Verification items for this drawing (mm, ordinates from the low corner). Round coordinates to 2 decimals unless told otherwise and drop trailing zeros. Write each loop counter-clockwise with the first axis right and the second up, starting at its lowest first coordinate (ties: lowest second). Pieces come first, ordered by that corner, then holes.
Item 1: Cross-section at A-A (x = 8). Enter the section's corners in (y, z).
Item 2: Scan lines: probe 1 along Y at (x, z) = (15.5, 3.5); probe 2 along Z at (x, y) = (17.5, 7.5) (1 decimal); probe 3 along Y at (x, z) = (12.5, 5.75). Record each from-to range of solid material in increasing order.
Item 3: Depth check by flat-ended pin: P1, Ø2, axis at y = 6, z = 3.5, coming from the -X side; P2, Ø1.5, axis at x = 22.5, z = 5, coming from the -Y side; P3, Ø2, axis at x = 14, z = 1.5, coming from the +Y side. Enter the tip coordinate at first touch or a pass-through.
Item 4: Draft check along Z on the marked faces 1 and 2. Enter one of: pulls with the +Z half, pulls with the -Z half, needs draft (parallel to the pull), parting line crosses it, or undercut.
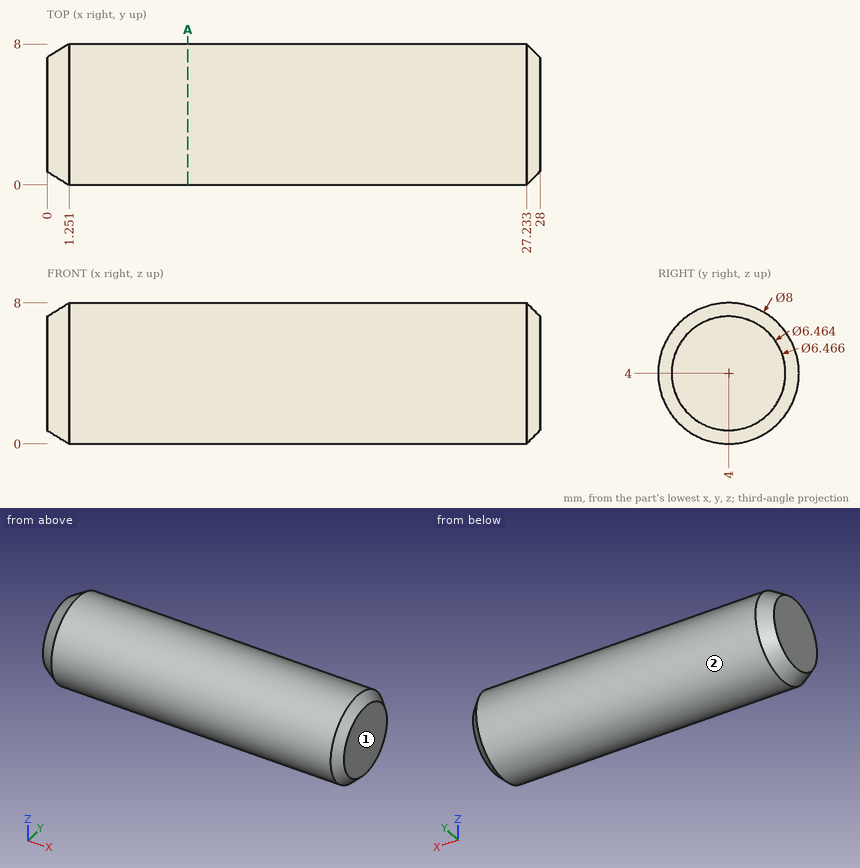
Resolved:
1. outline: circle Ø8 at (4, 4)
2. probe 1: y = 0.03 to 7.97
2. probe 2: z = 2.1 to 5.9
2. probe 3: y = 0.4 to 7.6
3. P1: stops at x = 0
3. P2: stops at y = 0.01
3. P3: stops at y = 7.71
4. face 1: needs draft
4. face 2: parting line crosses it
